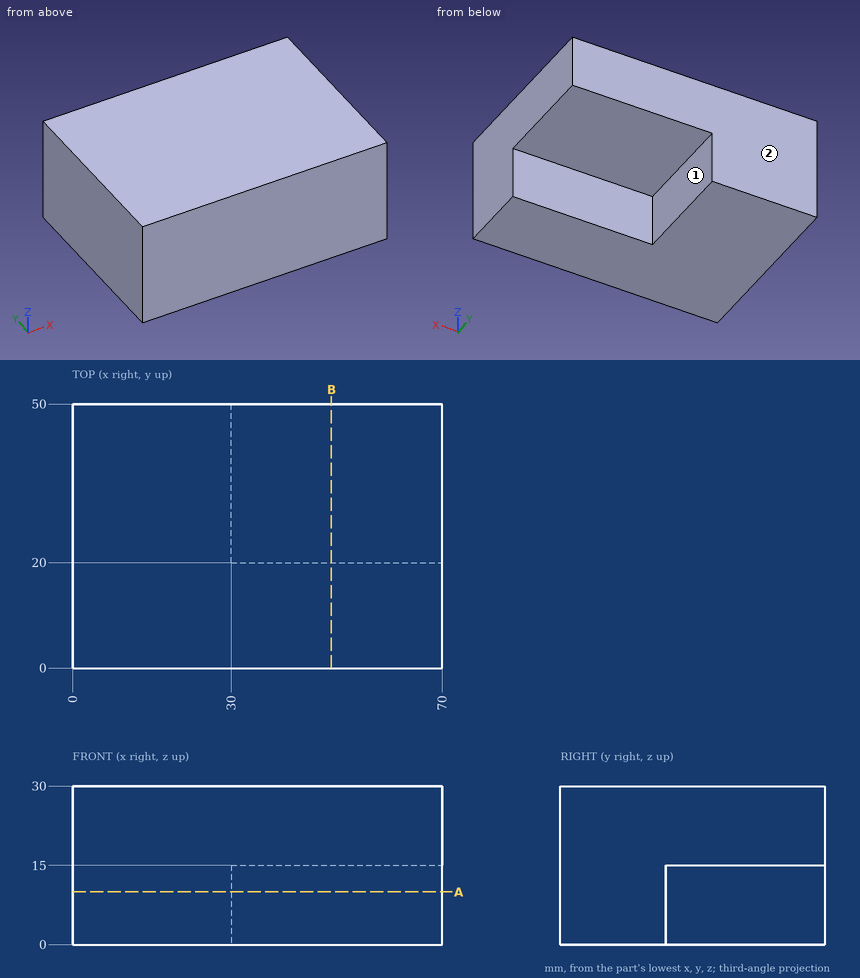
Print and shaded views of the part. All mm, measured from the part's lowest x, y and z. A direction names the side the tool comes from. Coordinates: 2 decimals unless noted, no trailing zeros. Write each loop counter-clockwise with the first axis right and the second up, starting at its lowest first coordinate (ties: lowest second). Pieces come first, ordered by that corner, then holes. Notation, with made-up numbers: (39, -4) - (64, -4) arc R33 ccw to (64, 25) - close; hole circle Ø4 at (35, 62). An arc over 180 degrees is marked (long way). One line per question, with ' | ' between items. Start each with the question number.
Q1. Cut at B-B, the plane x = 49. List the corners of the cut face in (y, z).
Q2. 3-axis set-ups, long thin cutter, end or side, ignore diameter. For the marked faces 1 and 2: which of +Z, -Z, +X, -X, +Y, -Y reach the whole face in a straight line?
Q3. Pin check, flat tips, straight feed: pin 1 (5 mm diameter, centred on y = 27.5, z = 5, fed in from +X); pin 2 (2 mm diameter, centred on x = 34, y = 25.5, fed in from -Z); pin 3 (12 mm diameter, centred on x = 50, z = 6.5, fed in from +Y). Stop position of each tip, or through.
Q4. Drill centre lines: line 1 (Y direction, x = 34, z = 11); line 2 (X direction, y = 40, z = 7); line 3 (Z direction, x = 56, y = 35). Where is each one in solid material? Low to high. Write a range as [from, to].
Q5. Cut at A-A, the plane z = 10. List the corners of the cut face in (x, y).
Answer below:
1) outline: (0, 0) - (20, 0) - (20, 15) - (50, 15) - (50, 30) - (0, 30) - close
2) face 1: -Z, +X, +Y | face 2: +Z, -Z, +X, -X, +Y
3) pin 1: x = 30 | pin 2: z = 15 | pin 3: y = 20
4) line 1: [0, 20] | line 2: [0, 30] | line 3: [15, 30]
5) outline: (0, 0) - (70, 0) - (70, 20) - (30, 20) - (30, 50) - (0, 50) - close
